Build history of the part. All positions in model axes, mm. Face numbers are marked on the shaded views. A direction names the side the tool comes from. Round coordinates to 2 decimals unless told otherwise and drop trailing zeros. Loops run counter-clockwise (first coordinate to the right, second up) from the corner with the lowest first, then second, coordinate; pieces in that order, holes last. Notation, with made-up numbers: (79, 17.25) - (108, 17.25) arc R15 cw to (108, 33.25) - close; hole circle Ø1 at (79, -16.75). An arc over 180 degrees is marked (long way). Use one line per item in the form item = value. Start each with the question number.
Q1. Saw through at B-B (x = 26). Give the cut face in (y, z).
Q2. Drill centre lines: line 1 (X direction, y = 24.15, z = -16); line 2 (Y direction, x = -16, z = 2.5); line 3 (X direction, y = 6.5, z = -3). Where is each one in solid material? Low to high.
Q3. Saw through at A-A (z = 16). Give the cut face in (x, y).
Q4. Pin check, flat tips, straight feed: pin 1 (1.5 mm diameter, centred on x = -21.5, z = -4.5, fed in from -Y); pin 2 (3 mm diameter, centred on x = -4, y = 12, fed in from +Z); pin 3 (12 mm diameter, centred on x = 9, y = 11.5, fed in from +Z); pin 4 (1.8 mm diameter, centred on x = -26, z = -16, fed in from -Y). Stop position of each tip, or through.
Q5. 3-axis set-ups, long thin cutter, end or side, ignore diameter. For the marked faces 1 and 2: which of +Z, -Z, +X, -X, +Y, -Y reach the whole face in a straight line?
Q6. Saw through at C-C (x = 0). Give the cut face in (y, z), then the cut area to 3 significant figures.
Q7. Saw through at D-D (z = 0). Give the cut face in (x, y).
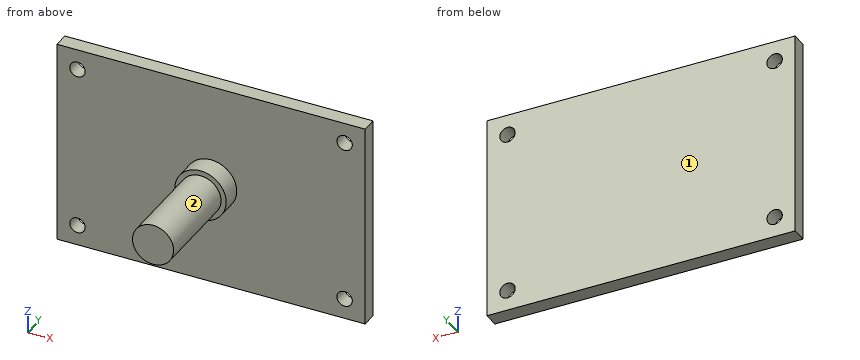
```python
from build123d import *

# Parameters (mm, degrees)
SKETCH1_R           = 4
BOSS_EXTRUDE1_DEPTH = 18
SKETCH2_R           = 5
BOSS_EXTRUDE2_DEPTH = 4
SKETCH3_W           = 60
SKETCH3_H           = 40
SKETCH3_R           = 1.5
BOSS_EXTRUDE3_DEPTH = 3


with BuildPart() as part:
    # Sketch1 → Boss-Extrude1 (new body)
    with BuildSketch(Plane(origin=(0, 0, 0), x_dir=(1, 0, 0), z_dir=(0, 1, 0))):
        with Locations(Location((0, 0, 0), (0, 0, 270))):
            Circle(SKETCH1_R)
    extrude(amount=BOSS_EXTRUDE1_DEPTH)

    # Sketch2 → Boss-Extrude2 (add)
    with BuildSketch(Plane(origin=(0, 18, 0), x_dir=(1, 0, 0), z_dir=(0, 1, 0))):
        with Locations(Location((0, 0, 0), (0, 0, 270))):
            Circle(SKETCH2_R)
    extrude(amount=BOSS_EXTRUDE2_DEPTH)

    # Sketch3 → Boss-Extrude3 (add)
    with BuildSketch(Plane(origin=(0, 22, 0), x_dir=(1, 0, 0), z_dir=(0, 1, 0))):
        Rectangle(SKETCH3_W, SKETCH3_H)
        with Locations(Location((-26, 16, 0), (0, 0, 270))):
            Circle(SKETCH3_R, mode=Mode.SUBTRACT)
        with Locations(Location((26, 16, 0), (0, 0, 90))):
            Circle(SKETCH3_R, mode=Mode.SUBTRACT)
        with Locations(Location((26, -16, 0), (0, 0, 270))):
            Circle(SKETCH3_R, mode=Mode.SUBTRACT)
        with Locations(Location((-26, -16, 0), (0, 0, 90))):
            Circle(SKETCH3_R, mode=Mode.SUBTRACT)
    extrude(amount=BOSS_EXTRUDE3_DEPTH)


solid = part.part
```
Report:
q1.outline = (22, -20) - (25, -20) - (25, -17.5) - (22, -17.5) - close; (22, -14.5) - (25, -14.5) - (25, 14.5) - (22, 14.5) - close; (22, 17.5) - (25, 17.5) - (25, 20) - (22, 20) - close
q2.line_1 = -30 to -27.5, -24.5 to 24.5, 27.5 to 30
q2.line_2 = 22 to 25
q2.line_3 = -2.65 to 2.65
q3.outline = (-30, 22) - (-27.5, 22) - (-27.5, 25) - (-30, 25) - close; (-24.5, 22) - (24.5, 22) - (24.5, 25) - (-24.5, 25) - close; (27.5, 22) - (30, 22) - (30, 25) - (27.5, 25) - close
q4.pin_1 = 22
q4.pin_2 = 3.12
q4.pin_3 = 2.65
q4.pin_4 = through
q5.face_1 = +Z, -Z, +X, -X, +Y
q5.face_2 = -Y
q6.outline = (0, -4) - (18, -4) - (18, -5) - (22, -5) - (22, -20) - (25, -20) - (25, 20) - (22, 20) - (22, 5) - (18, 5) - (18, 4) - (0, 4) - close
q6.area = 304 mm²
q7.outline = (-30, 22) - (-5, 22) - (-5, 18) - (-4, 18) - (-4, 0) - (4, 0) - (4, 18) - (5, 18) - (5, 22) - (30, 22) - (30, 25) - (-30, 25) - close
